Could you check a few things on this drawing? It's one solid part, dimensions in mm from its lowest x, y, z. A direction names the side the tool comes from. Round coordinates to 2 decimals unless told otherwise and drop trailing zeros. Loops run counter-clockwise (first coordinate to the right, second up) from the corner with the lowest first, then second, coordinate; pieces in that order, holes last.
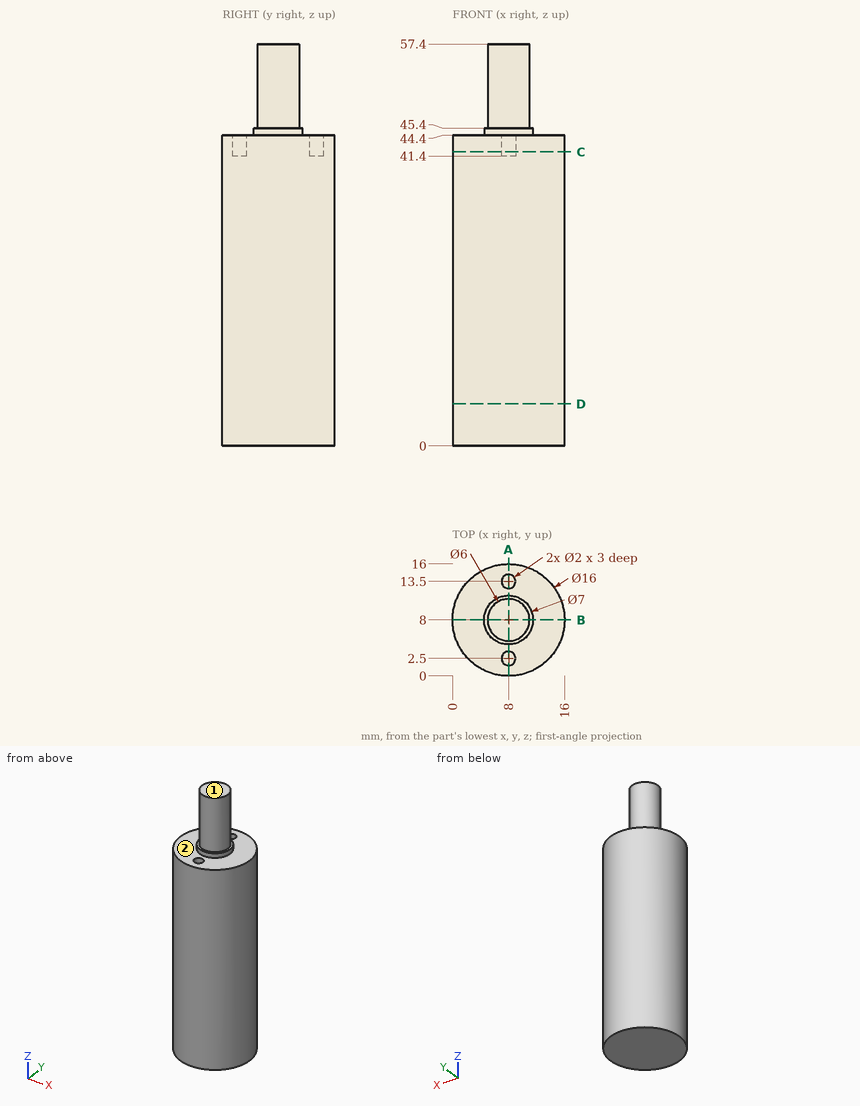
(1) Which directions (+Z, -Z, +X, -X, +Y, -Y) give clear straight access to the entire face, cutting with the end or side of a thin tool? Please do the marked faces 1 and 2.
(2) If I drill on line 1 (Y direction, x = 8, z = 42.8); line 2 (Z direction, x = 2, y = 9.25); line 3 (Y direction, x = 14, z = 13.5), over which ranges is the centre line in solid material (lowest first)?
(3) Suppose I cut it at D-D (z = 6). Write out the boundary of the cut face in (x, y), then the cut area to 3 significant figures.
(4) Suppose I cut it at A-A (x = 8). Write out the boundary of the cut face in (y, z).
(5) For pin 1 (2 mm diameter, centred on x = 8.5, y = 2.5, fed in from +Z); pin 2 (5 mm diameter, centred on x = 3, z = 37, fed in from -Y), each with a flat end and sliding along its axis, tell me the tip position at first contact or that it passes through.
(6) Suppose I cut it at C-C (z = 42). Write out the boundary of the cut face in (x, y).
(7) Suppose I cut it at B-B (y = 8). Write out the boundary of the cut face in (x, z).
Check result:
1. face 1: +Z, +X, -X, +Y, -Y
1. face 2: +Z
2. line 1: y = 0 to 1.5, 3.5 to 12.5, 14.5 to 16
2. line 2: z = 0 to 44.4
2. line 3: y = 2.71 to 13.29
3. outline: circle Ø16 at (8, 8)
3. area: 201 mm2
4. outline: (0, 0) - (16, 0) - (16, 44.4) - (14.5, 44.4) - (14.5, 41.4) - (12.5, 41.4) - (12.5, 44.4) - (11.5, 44.4) - (11.5, 45.4) - (11, 45.4) - (11, 57.4) - (5, 57.4) - (5, 45.4) - (4.5, 45.4) - (4.5, 44.4) - (3.5, 44.4) - (3.5, 41.4) - (1.5, 41.4) - (1.5, 44.4) - (0, 44.4) - close
5. pin 1: stops at z = 44.4
5. pin 2: stops at y = 0.4
6. outline: circle Ø16 at (8, 8); hole circle Ø2 at (8, 2.5); hole circle Ø2 at (8, 13.5)
7. outline: (0, 0) - (16, 0) - (16, 44.4) - (11.5, 44.4) - (11.5, 45.4) - (11, 45.4) - (11, 57.4) - (5, 57.4) - (5, 45.4) - (4.5, 45.4) - (4.5, 44.4) - (0, 44.4) - close
